Could you check a few things on this model? Use its own coordinates, in mm. A direction names the side the tool comes from. Give positions to 0.01 mm unless a question says otherwise; leave off trailing zeros. Loops run counter-clockwise (first coordinate to the right, second up) from the corner with the lowest first, then second, coordinate; pieces in that order, holes last. Notation, with made-up numbers: (34.5, 78) - (56.5, 78) arc R18 ccw to (56.5, 83) - close; hole circle Ø6 at (-10, -13). An arc over 180 degrees is marked (long way). Write each question's results on one line, items separated by ' | '. Start each with the question number.
1) On a 3-axis mill with a long thin cutter (end or side, diameter ignored), from which of +Z, -Z, +X, -X, +Y, -Y can I reach the whole of each face in a straight line? I mean faces 1 (the face through (0, 0, -10)), 2 (the face through (-1.4, 0, 0)), 3 (the face through (0, -1, 2)). Say none if no direction works.
2) If we mould it in two halves opening along X, with no side actions, what happens to faces 4 (the face through (-0.87, -0.49, 1.82)), 5 (the face through (-2.579, 1.978, 0.951)), 6 (the face through (1, 1, 2.5))? For each: +X half, -X half, draft (parallel to the pull), parting line (faces both ways), or undercut.
3) If I drill on probe 1 along X at (y, z) = (0, -5); probe 2 along Z at (x, y) = (-1.75, 0.5); probe 3 along Z at (x, y) = (-0.5, 0.25) (3 decimals), over which ranges is the centre line in solid material (lowest first)? Write a range as [from, to].
4) I want a section at B-B, the plane z = -7.75. Write out the boundary of the cut face in (x, y).
5) I want a section at A-A, the plane x = 0. Write out the boundary of the cut face in (y, z) (3 decimals).
6) I'm going to push flat-ended pins straight in: pin 1 (3 mm diameter, centred on y = -1, z = -3.5, fed in from -X); pin 2 (1 mm diameter, centred on x = -1.5, z = -6.5, fed in from +Y). Where does each tip first touch, or does it pass through?
from build123d import *

# Parameters (mm, degrees)
SHANK_TIP_CHAMFER_SIZE = 0.3
PAN_HEAD_ROUND_R       = 0.625
HEX_DRIVE_CUT_DEPTH    = 1.375


with BuildPart() as part:
    # Screw Section → Screw Blank Revolve (revolve)
    with BuildSketch(Plane(origin=(0, 0, 0), x_dir=(1, 0, 0), z_dir=(0, 1, 0))):
        Polygon((0, 10), (1.2, 10), (1.2, 0), (3.25, 0), (3.25, -2.5), (0, -2.5), align=None)
    revolve(axis=Axis((0, 0, 10.123), (0, 0, -1)))

    # Shank Tip Chamfer
    shank_tip_chamfer_edges = [part.edges().sort_by_distance(p)[0] for p in [
        (-1.2, 0, -10),
    ]]
    chamfer(shank_tip_chamfer_edges, length=SHANK_TIP_CHAMFER_SIZE)

    # Pan Head Round
    pan_head_round_edges = [part.edges().sort_by_distance(p)[0] for p in [
        (-3.25, 0, 2.5),
    ]]
    fillet(pan_head_round_edges, radius=PAN_HEAD_ROUND_R)

    # Hex Drive Sketch → Hex Drive Cut (cut)
    with BuildSketch(Plane.XY.offset(2.5)):
        Polygon((1.154700538, 0), (0.577350269, 1), (-0.577350269, 1), (-1.154700538, 0), (-0.577350269, -1), (0.577350269, -1), align=None)
    extrude(amount=-HEX_DRIVE_CUT_DEPTH, mode=Mode.SUBTRACT)


solid = part.part
Answers:
1) face 1: -Z, +X, -X, +Y, -Y | face 2: -Z | face 3: +Z
2) face 4: undercut | face 5: parting line | face 6: draft
3) probe 1: x = [-1.2, 1.2] | probe 2: z = [0, 2.5] | probe 3: z = [-10, 1.125]
4) outline: circle Ø2.4 at (0, 0)
5) outline: (-3.25, 0) - (-1.2, 0) - (-1.2, -9.7) - (-0.9, -10) - (0.9, -10) - (1.2, -9.7) - (1.2, 0) - (3.25, 0) - (3.25, 1.875) arc R0.625 ccw to (2.625, 2.5) - (1, 2.5) - (1, 1.125) - (-1, 1.125) - (-1, 2.5) - (-2.625, 2.5) arc R0.625 ccw to (-3.25, 1.875) - close
6) pin 1: stops at x = -1.2 | pin 2: stops at y = 0.66
